Build history of the part. All positions in model axes, mm. A direction names the side the tool comes from. Round coordinates to 2 decimals unless told otherwise and drop trailing zeros. Write each loop counter-clockwise with the first axis right and the second up, starting at its lowest first coordinate (ties: lowest second). Pieces come first, ordered by that corner, then holes.
1) Saw through at C-C (y = 17.5). Write the cut outline in (x, z), plus the area to 3 significant figures.
2) Which spindle directions (+Z, -Z, +X, -X, +Y, -Y) get a long thin tool onto all of the face, cutting with end or side? Do faces 1 (the flat face through (0, 107.95, 0)), 2 (the flat face through (0, 98, -4.762)), 3 (the flat face through (0, 98, 4.762)), 4 (the flat face through (0, 10, -4.762)), 5 (the cylindrical face through (-1.707, 104.277, -0.067)). Say none if no direction does.
3) Saw through at D-D (y = 68). Write the cut outline in (x, z), plus the area to 3 significant figures.
4) Saw through at A-A (x = 0). State how many separate pieces and enclosed holes the cut face has, plus the area to 3 significant figures.
5) Flat gauge pins, fed straight in: pin 1 (10 mm diameter, centred on x = 0, y = 6.35, fed in from +Z); pin 2 (2 mm diameter, centred on x = 9, z = -9, fed in from +Y); pin 3 (1.5 mm diameter, centred on x = -7, z = 9.5, fed in from -Y); pin 4 (4 mm diameter, centred on x = 0, y = 101.6, fed in from -Z). Where does each tip first touch, or does it go through?
6) Pull direction Y, two halves, no side cores. Call faces 6 (the flat face through (0, 12, 4.762)), 7 (the cylindrical face through (-1.707, 9.027, -0.067)), 8 (the cylindrical face through (0.16, 83.15, -6.14)): +Y half, -Y half, draft (parallel to the pull), parting line (faces both ways), or undercut.
7) Wall check: probe 1 along Y at (x, z) = (0, -0.5) (3 decimals); probe 2 along Y at (x, z) = (2.25, 3.5); probe 3 along Z at (x, y) = (-6, 89). Give the ranges that are in metal, low to high.
from build123d import *

# Parameters (mm, degrees)
SKETCH1_R           = 12.7
BOSS_EXTRUDE1_DEPTH = 107.95
SKETCH2_W           = 7.9375
SKETCH2_H           = 31.75
CUT_EXTRUDE1_DEPTH  = 112.622813528
FILLET1_R           = 12.7
MIRROR1_START       = -11.773215198
MIRROR1_DEPTH       = 23.546430296
HOLE1_D             = 6.35
FILLET6_R           = 6.35


# Read off the part's stored shape, not the designer's step: Mirror1
with BuildPart() as part:
    # Sketch1 → Boss-Extrude1 (new body)
    with BuildSketch(Plane(origin=(0, 0, 0), x_dir=(1, 0, 0), z_dir=(0, 1, 0))):
        with Locations(Location((0, 0, 0), (0, 0, 270))):
            Circle(SKETCH1_R)
    extrude(amount=BOSS_EXTRUDE1_DEPTH)

    # Sketch2 → Cut-Extrude1 (cut, through all)
    with BuildSketch(Plane(origin=(12.7, 0, 0), x_dir=(0, 0, -1), z_dir=(1, 0, 0))):
        with Locations((8.73125, 92.075)):
            Rectangle(SKETCH2_W, SKETCH2_H)
        with Locations((-8.73125, 92.075)):
            Rectangle(SKETCH2_W, SKETCH2_H)
    extrude(amount=-CUT_EXTRUDE1_DEPTH, mode=Mode.SUBTRACT)

    # Fillet1
    # the kernel refuses this fillet: 12.7 mm, written as the material it adds along each edge
    with BuildSketch(Plane(origin=(43.523215098, 76.2, 4.7625), x_dir=(0, 1, 0), z_dir=(-1, 0, 0))) as fillet1_piece_1_section:
        with BuildLine():
            CenterArc((FILLET1_R, -FILLET1_R), FILLET1_R, 90, 90)
            Line((0, -FILLET1_R), (0, 0))
            Line((0, 0), (FILLET1_R, 0))
        make_face()
    fillet1_piece_1 = extrude(amount=87.046430197, mode=Mode.PRIVATE)
    fillet1_piece_1 = fillet1_piece_1 & Plane(origin=(0, 79.544884305, 0), x_dir=(0, 0, 1), z_dir=(0, -1, 0)) * Cylinder(12.7, 225, mode=Mode.PRIVATE)
    add(fillet1_piece_1)
    with BuildSketch(Plane(origin=(43.523215098, 76.2, -4.7625), x_dir=(0, 0, -1), z_dir=(-1, 0, 0))) as fillet1_piece_2_section:
        with BuildLine():
            CenterArc((FILLET1_R, -FILLET1_R), FILLET1_R, 90, 90)
            Line((0, -FILLET1_R), (0, 0))
            Line((0, 0), (FILLET1_R, 0))
        make_face()
    fillet1_piece_2 = extrude(amount=87.046430197, mode=Mode.PRIVATE)
    fillet1_piece_2 = fillet1_piece_2 & Plane(origin=(0, 79.544821944, 0), x_dir=(0, 0, 1), z_dir=(0, -1, 0)) * Cylinder(12.7, 225, mode=Mode.PRIVATE)
    add(fillet1_piece_2)

    # Mirror1 outline → Mirror1 (cut)
    with BuildSketch(Plane.YZ.offset(MIRROR1_START)):
        with BuildLine():
            Line((19.05, -4.7625), (0, -4.7625))
            Line((0, -4.7625), (0, -14))
            Line((0, -14), (31.349026101, -14))
            Line((31.349026101, -14), (30.823419426, -12.700505142))
            ThreePointArc((30.823419426, -12.700505142), (26.149741731, -6.932368598), (19.05, -4.7625))
        make_face()
        with BuildLine():
            Line((0, 14), (0, 4.7625))
            Line((0, 4.7625), (19.05, 4.7625))
            ThreePointArc((19.05, 4.7625), (26.149741731, 6.932368598), (30.823419426, 12.700505142))
            Line((30.823419426, 12.700505142), (31.349026101, 14))
            Line((31.349026101, 14), (0, 14))
        make_face()
    extrude(amount=MIRROR1_DEPTH, mode=Mode.SUBTRACT)

    # Hole1 (through all)
    with Locations(Plane.XY.offset(4.7625)):
        with Locations((0, 101.6), (0, 6.35)):
            Hole(HOLE1_D / 2)

    # Fillet6
    # the kernel refuses this fillet: 6.35 mm, written as the material it takes off along each edge
    with BuildSketch(Plane(origin=(0, 107.95, 0), x_dir=(-0.06367759150342109, 0, 0.9979705227812711), z_dir=(-0.9979705227812711, 0, -0.06367759150342109))) as fillet6_piece_1:
        with BuildLine():
            CenterArc((12.7 - FILLET6_R, -FILLET6_R), FILLET6_R, 0, 90)
            Line((12.7 - FILLET6_R, 0), (12.7, 0))
            Line((12.7, 0), (12.7, -FILLET6_R))
        make_face()
    revolve(axis=Axis((0, 107.95, 0), (0, 1, 0)), revolution_arc=187.301854803, mode=Mode.SUBTRACT)
    with BuildSketch(Plane(origin=(0, 0, 0), x_dir=(0.06367758856259068, 0, -0.9979705229689169), z_dir=(0.9979705229689169, 0, 0.06367758856259068))) as fillet6_piece_2:
        with BuildLine():
            CenterArc((12.7 - FILLET6_R, FILLET6_R), FILLET6_R, 270, 90)
            Line((12.7 - FILLET6_R, 0), (12.7, 0))
            Line((12.7, 0), (12.7, FILLET6_R))
        make_face()
    revolve(axis=Axis((0, 0, 0), (0, 1, 0)), revolution_arc=187.301854466, mode=Mode.SUBTRACT)
    with BuildSketch(Plane(origin=(0, 107.95, 0), x_dir=(0.06367759150341921, 0, -0.9979705227812712), z_dir=(0.9979705227812712, 0, 0.06367759150341921))) as fillet6_piece_3:
        with BuildLine():
            CenterArc((12.7 - FILLET6_R, -FILLET6_R), FILLET6_R, 0, 90)
            Line((12.7 - FILLET6_R, 0), (12.7, 0))
            Line((12.7, 0), (12.7, -FILLET6_R))
        make_face()
    revolve(axis=Axis((0, 107.95, 0), (0, 1, 0)), revolution_arc=187.301854803, mode=Mode.SUBTRACT)
    with BuildSketch(Plane(origin=(0, 0, 0), x_dir=(-0.06367759151119771, 0, 0.9979705227807748), z_dir=(-0.9979705227807748, 0, -0.06367759151119771))) as fillet6_piece_4:
        with BuildLine():
            CenterArc((12.7 - FILLET6_R, FILLET6_R), FILLET6_R, 270, 90)
            Line((12.7 - FILLET6_R, 0), (12.7, 0))
            Line((12.7, 0), (12.7, FILLET6_R))
        make_face()
    revolve(axis=Axis((0, 0, 0), (0, 1, 0)), revolution_arc=187.301854804, mode=Mode.SUBTRACT)


solid = part.part
Evaluation:
1. outline: (-11.77, -4.76) - (11.77, -4.76) arc R12.7 ccw to (11.77, 4.76) - (-11.77, 4.76) arc R12.7 ccw to start
1. area: 236 mm2
2. face 1: +Z, -Z, +X, -X, +Y
2. face 2: -Z, +X, -X, +Y
2. face 3: +Z, +X, -X, +Y
2. face 4: -Z, +X, -X, -Y
2. face 5: +Z, -Z
3. outline: circle Ø25.4 at (0, 0)
3. area: 507 mm2
4. separate pieces: 3
4. enclosed holes: 0
4. area: 1,750 mm2
5. pin 1: stops at z = 4.76
5. pin 2: stops at y = 80.43
5. pin 3: stops at y = 28.29
5. pin 4: passes through
6. face 6: draft
6. face 7: undercut
6. face 8: +Y half
7. probe 1: y = 0 to 3.175, 9.525 to 98.425, 104.775 to 107.95
7. probe 2: y = 0 to 4.11, 8.59 to 99.36, 103.84 to 107.95
7. probe 3: z = -4.76 to 4.76
